```python
from build123d import *

# Parameters (mm, degrees)
BOSS_EXTRUDE1_DEPTH = 15
SKETCH2_W           = 10
SKETCH2_H           = 2.5
SKETCH2_H_2         = 7.5
CUT_EXTRUDE2_DEPTH  = 17.5


with BuildPart() as part:
    # Sketch1 → Boss-Extrude1 (new body)
    with BuildSketch(Plane.XY):
        Polygon((0, 0), (0, 20), (10, 20), (20, 10), (20, 0), align=None)
    extrude(amount=BOSS_EXTRUDE1_DEPTH)

    # Sketch2 → Cut-Extrude2 (cut)
    with BuildSketch(Plane(origin=(20, 0, 0), x_dir=(0, 0, -1), z_dir=(1, 0, 0))):
        with Locations((-7.5, 18.75)):
            Rectangle(SKETCH2_W, SKETCH2_H)
        with Locations((-7.5, 13.75)):
            Rectangle(SKETCH2_W, SKETCH2_H_2)
        with Locations((-7.5, 6.25)):
            Rectangle(SKETCH2_W, SKETCH2_H_2)
    extrude(amount=-CUT_EXTRUDE2_DEPTH, mode=Mode.SUBTRACT)


solid = part.part
```
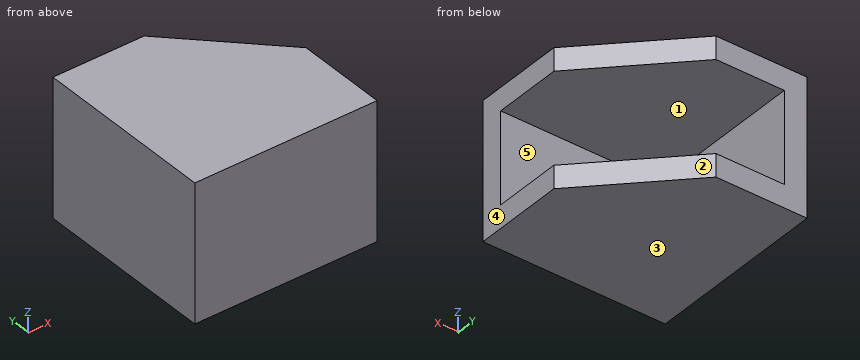
Part model, mm, in its own coordinate system. Face numbers are marked on the shaded views. A direction names the side the tool comes from. Round coordinates to 2 decimals unless told otherwise and drop trailing zeros. Loops run counter-clockwise (first coordinate to the right, second up) from the corner with the lowest first, then second, coordinate; pieces in that order, holes last.
1. Drill centre lines: line 1 along Z through (x, y) = (11.5, 7.5); line 2 along X through (y, z) = (5, 7.25). Where is each one in solid material? Low to high.
Solutions:
line 1: z = 0 to 2.5, 12.5 to 15
line 2: x = 0 to 2.5
2. Slice it at D-D (z = 1.25). Give the cut face in (x, y).
Solutions:
outline: (0, 0) - (20, 0) - (20, 10) - (10, 20) - (0, 20) - close
3. Slice it at C-C (z = 3.5). Give the cut face in (x, y).
Solutions:
outline: (0, 0) - (20, 0) - (20, 2.5) - (2.5, 2.5) - (2.5, 20) - (0, 20) - close
4. Slice it at A-A (y = 9.5). Give the cut face in (x, z), and give its area (3 significant figures).
Solutions:
outline: (0, 0) - (20, 0) - (20, 2.5) - (2.5, 2.5) - (2.5, 12.5) - (20, 12.5) - (20, 15) - (0, 15) - close
area: 125 mm2
5. 3-axis set-ups, long thin cutter, end or side, ignore diameter. For the marked faces 4 and 5: which of +Z, -Z, +X, -X, +Y, -Y reach the whole face in a straight line?
Solutions:
face 4: +Z, -Z, +X, +Y, -Y
face 5: +X, +Y
6. Flat gauge pins, fed straight in: pin 1 (3 mm diameter, centred on x = 14, z = 7.5, fed in from +Y); pin 2 (1.5 mm diameter, centred on y = 15, z = 4.5, fed in from +X). Where does each tip first touch, or does it go through?
Solutions:
pin 1: stops at y = 2.5
pin 2: stops at x = 2.5
7. Slice it at B-B (x = 13.5). Give the cut face in (y, z), and give its area (4 significant figures).
Solutions:
outline: (0, 0) - (16.5, 0) - (16.5, 2.5) - (2.5, 2.5) - (2.5, 12.5) - (16.5, 12.5) - (16.5, 15) - (0, 15) - close
area: 107.5 mm2
8. Two-plate mould, pull along Z, no slides. Class the marked faces 1, 2 and 3: pulls with the +Z half, pulls with the -Z half, needs draft (parallel to the pull), parting line crosses it, or undercut.
Solutions:
face 1: undercut
face 2: needs draft
face 3: pulls with the -Z half
